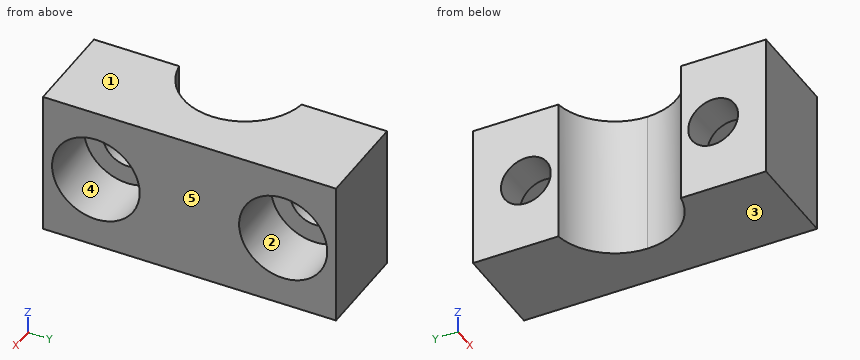
from build123d import *

# Parameters (mm, degrees)
F1_DEPTH = 9.6
F2_R     = 1.65
F3_DEPTH = 25
F2_R_2   = 2.9
F2_R_3   = 2.917698
F4_DEPTH = 4


with BuildPart() as f1:
    # F0 (on Top) → F1 (new body)
    with BuildSketch(Plane.XY):
        with BuildLine():
            ThreePointArc((-6.4, 13.75586), (-3.89597, 12.378619), (-2.9, 9.7))
            ThreePointArc((-2.9, 9.7), (-3.89597, 7.021381), (-6.4, 5.64414))
            Line((-6.4, 5.64414), (-6.4, 0))
            Line((-6.4, 0), (0, 0))
            Line((0, 0), (0, 19.4))
            Line((0, 19.4), (-6.4, 19.4))
            Line((-6.4, 19.4), (-6.4, 13.75586))
        make_face()
    extrude(amount=F1_DEPTH)

    # F2 (on Right) → F3 (cut)
    with BuildSketch(Plane.YZ):
        with Locations((3.5, 4.8)):
            Circle(F2_R)
        with Locations((15.9, 4.8)):
            Circle(F2_R)
    extrude(amount=-F3_DEPTH, mode=Mode.SUBTRACT)

    # F2 (on Right) → F4 (cut)
    with BuildSketch(Plane.YZ):
        with Locations((3.5, 4.8)):
            Circle(F2_R_2)
        with Locations((3.5, 4.8)):
            Circle(F2_R, mode=Mode.SUBTRACT)
        with Locations((15.9, 4.8)):
            Circle(F2_R_3)
        with Locations((15.9, 4.8)):
            Circle(F2_R, mode=Mode.SUBTRACT)
    extrude(amount=-F4_DEPTH, mode=Mode.SUBTRACT)


solid = f1.part
Geometry check sheet. Reference: the model listing, model coordinates, mm. Face numbers are marked on the shaded views. A direction names the side the tool comes from. Give positions to 0.01 mm unless a question says otherwise; leave off trailing zeros. Order: outer loops, then holes, each group sorted by start corner. A loop starts at its lowest first (then second) coordinate and runs counter-clockwise, first axis right, second up. Notation, with made-up numbers: (75.25, 7.25) - (106.25, 7.25) arc R12 cw to (106.25, 27.25) - close; hole circle Ø10 at (28.5, 54). An arc over 180 degrees is marked (long way). Use one line per item in the form item = value.
1) Sectioned sample at B-B (y = 15.9). Record the boundary of the cut face in (x, z), and give its area (3 significant figures).
Working result:
outline = (-6.4, 0) - (0, 0) - (0, 1.88) - (-4, 1.88) - (-4, 3.15) - (-6.4, 3.15) - close; (-6.4, 6.45) - (-4, 6.45) - (-4, 7.72) - (0, 7.72) - (0, 9.6) - (-6.4, 9.6) - close
area = 30.2 mm^2
2) Sectioned sample at C-C (x = -6). Record the boundary of the cut face in (y, z).
Working result:
outline = (0, 0) - (5.72, 0) - (5.72, 9.6) - (0, 9.6) - close; (13.68, 0) - (19.4, 0) - (19.4, 9.6) - (13.68, 9.6) - close; hole circle Ø3.3 at (3.5, 4.8); hole circle Ø3.3 at (15.9, 4.8)
3) Material ranges on probe 1 along Z at (x, y) = (-2.35, 3.5); probe 2 along Z at (x, y) = (-5.9, 3.5); probe 3 along Y at (x, z) = (-2.5, 7), recorded low to high. Write a range as from..to.
Working result:
probe_1 = 0..1.9, 7.7..9.6
probe_2 = 0..3.15, 6.45..9.6
probe_3 = 0..1.61, 5.39..13.98, 17.82..19.4
4) Draft check along Z on the marked faces 3, 4 and 5. Enter one of: released by +Z, released by -Z, zero draft, split by the parting line, or undercut.
Working result:
face_3 = released by -Z
face_4 = undercut
face_5 = zero draft
5) Access from +Z, -Z, +X, -X, +Y, -Y to the whole of each face (thin tool, end or side, straight path). Record for the marked faces 1 and 2.
Working result:
face_1 = +Z, +X, -X, +Y, -Y
face_2 = +X
6) Sectioned sample at A-A (z = 4.8). Record the boundary of the cut face in (x, y).
Working result:
outline = (-6.4, 0) - (0, 0) - (0, 0.6) - (-4, 0.6) - (-4, 1.85) - (-6.4, 1.85) - close; (-6.4, 5.15) - (-4, 5.15) - (-4, 6.4) - (0, 6.4) - (0, 12.98) - (-4, 12.98) - (-4, 14.25) - (-6.4, 14.25) - (-6.4, 13.76) arc R4.1 cw to (-2.9, 9.7) arc R4.1 cw to (-6.4, 5.64) - close; (-6.4, 17.55) - (-4, 17.55) - (-4, 18.82) - (0, 18.82) - (0, 19.4) - (-6.4, 19.4) - close
7) Sectioned sample at D-D (z = 8.5). Record the boundary of the cut face in (x, y), and give its area (3 significant figures).
Working result:
outline = (-6.4, 0) - (0, 0) - (0, 19.4) - (-6.4, 19.4) - (-6.4, 13.76) arc R4.1 cw to (-2.9, 9.7) arc R4.1 cw to (-6.4, 5.64) - close
area = 103 mm^2
8) Depth check by flat-ended pin: pin 1 Ø1.8 at (y, z) = (14.5, 5) entering from +X. Enter the tip coordinate at first touch or a pass-through.
Working result:
pin_1 = -4
